The listing builds one solid part. Answer for the finished solid, in the listing's coordinates (mm). Coordinates: 2 decimals unless noted, no trailing zeros. Order: outer loops, then holes, each group sorted by start corner. A loop starts at its lowest first (then second) coordinate and runs counter-clockwise, first axis right, second up. Notation, with made-up numbers: (-11.5, 86) - (33.5, 86) arc R22 ccw to (33.5, 117) - close; hole circle Ø8 at (75.25, -27). An arc over 180 degrees is marked (long way). Use a Markdown table: item, result. Add a question column.
Item 1: Find the intervals of material crossed by line 1 along Y through (x, z) = (0, 0.65); line 2 along Y through (x, z) = (27.5, 0.7); line 3 along X through (y, z) = (-0.5, 0.75), in increasing order.
Item 2: The part is cut by section D-D, the plane y = 0. Give the vertices of the cut face in (x, z), then the cut area to 3 significant figures.
Item 3: The part is cut by section C-C, the plane z = 0.4. Give the vertices of the cut face in (x, y), then the cut area to 3 significant figures.
Item 4: The part is cut by section A-A, the plane x = 0. Give the vertices of the cut face in (y, z), then the cut area to 3 significant figures.
Item 5: The part is cut by section B-B, the plane y = 24. Give the vertices of the cut face in (x, z), then the cut area to 3 significant figures.
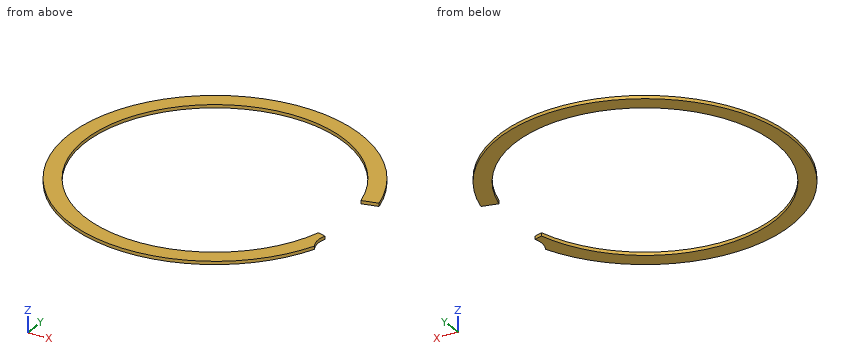
from build123d import *

# Parameters (mm, degrees)
BOSS_EXTRUDE1_DEPTH = 0.7874


with BuildPart() as part:
    # Sketch2 → Boss-Extrude1 (new body)
    with BuildSketch(Plane.XY):
        with BuildLine():
            Line((31.171102562, 8.352271759), (33.109329325, 8.871618055))
            Line((33.109329325, 8.871618055), (35.047556088, 9.390964351))
            ThreePointArc((35.047556088, 9.390964351), (-36.211242798, 2.295058655), (33.581480457, -13.740653898))
            ThreePointArc((33.581480457, -13.740653898), (32.810406003, -11.358014898), (33.109329325, -8.871618055))
            Line((33.109329325, -8.871618055), (31.171102562, -8.352271759))
            ThreePointArc((31.171102562, -8.352271759), (-32.2707, 0), (31.171102562, 8.352271759))
        make_face()
    extrude(amount=BOSS_EXTRUDE1_DEPTH)


solid = part.part
Solution:
| question | item | result |
|---|---|---|
| 1 | line 1 | y = -36.28 to -32.27, 32.27 to 36.28 |
| 1 | line 2 | y = -23.67 to -16.89, 16.89 to 23.67 |
| 1 | line 3 | x = -36.28 to -32.27 |
| 2 | outline | (-36.28, 0) - (-32.27, 0) - (-32.27, 0.79) - (-36.28, 0.79) - close |
| 2 | area | 3.16 mm2 |
| 3 | outline | (31.17, -8.35) arc R32.27 cw (long way) to (31.17, 8.35) - (35.05, 9.39) arc R36.28 ccw (long way) to (33.58, -13.74) arc R5.83 cw to (33.11, -8.87) - close |
| 3 | area | 786 mm2 |
| 4 | outline | (-36.28, 0) - (-32.27, 0) - (-32.27, 0.79) - (-36.28, 0.79) - close; (32.27, 0) - (36.28, 0) - (36.28, 0.79) - (32.27, 0.79) - close |
| 4 | area | 6.32 mm2 |
| 5 | outline | (-27.21, 0) - (-21.57, 0) - (-21.57, 0.79) - (-27.21, 0.79) - close; (21.57, 0) - (27.21, 0) - (27.21, 0.79) - (21.57, 0.79) - close |
| 5 | area | 8.88 mm2 |
